```python
from build123d import *

# Parameters (mm, degrees)
BOSS_EXTRUDE2_DEPTH = 8
CUT_EXTRUDE5_DEPTH  = 18.5
BOSS_EXTRUDE7_DEPTH = 8
SKETCH9_R           = 3.15
CUT_EXTRUDE6_DEPTH  = 8
CUT_EXTRUDE8_DEPTH  = 8
BOSS_EXTRUDE8_DEPTH = 8
SKETCH14_R          = 5
CUT_EXTRUDE10_DEPTH = 10
SKETCH15_R          = 6
CUT_EXTRUDE11_DEPTH = 4
SKETCH2_R           = 3.15
CUT_EXTRUDE12_DEPTH = 48


with BuildPart() as part:
    # Sketch1 → Boss-Extrude2 (new body)
    with BuildSketch(Plane(origin=(0, 0, 0), x_dir=(1, 0, 0), z_dir=(0, 1, 0))):
        Polygon((-36.064195387, 30.19821093), (-36.064195387, 45.055140387), (-24.456215945, 60.508200645), (25.928290152, 75.028423128), (63.192701615, 49.978777876), (57.8600206, 4.654046233), (5.024212079, -12.575443702), (-26.79369062, -0.934399252), align=None)
    extrude(amount=BOSS_EXTRUDE2_DEPTH)

    # Sketch7 → Cut-Extrude5 (cut)
    with BuildSketch(Plane(origin=(0, 8, 0), x_dir=(1, 0, 0), z_dir=(0, 1, 0))):
        Polygon((-23.90080129, 101.032848336), (-57.901406204, 20.736967462), (-18.158957139, -32.533824917), (87.924213713, -9.961236853), (85.311975199, 49.315634488), align=None)
        Polygon((-40.820623888, 23.42964982), (-5.371906334, -12.019067733), (42.940552226, -17.400063196), (73.057764711, 41.083606285), (-8.197554073, 82.927487203), align=None, mode=Mode.SUBTRACT)
    extrude(amount=-CUT_EXTRUDE5_DEPTH, mode=Mode.SUBTRACT)

    # Sketch8 → Boss-Extrude7 (add)
    with BuildSketch(Plane(origin=(0, 8, 0), x_dir=(1, 0, 0), z_dir=(0, 1, 0))):
        Polygon((-8.197554073, 82.927487203), (-40.820623888, 23.42964982), (-5.371906334, -12.019067733), (42.940552226, -17.400063196), (73.057764711, 41.083606285), align=None)
        Polygon((7.41963674, 62.005546744), (-9.746922841, 64.747246038), (-32.401642497, 23.42964982), (0, -4.674812176), (46.197479834, 11.841771544), (56.025503799, 35.943618774), align=None, mode=Mode.SUBTRACT)
    extrude(amount=-BOSS_EXTRUDE7_DEPTH)

    # Sketch9 → Cut-Extrude6 (cut)
    with BuildSketch(Plane(origin=(0, 0, 0), x_dir=(-1, 0, 0), z_dir=(0, -1, 0))):
        with Locations((-28.941808693, 3.473889793)):
            Circle(SKETCH9_R)
    extrude(amount=-CUT_EXTRUDE6_DEPTH, mode=Mode.SUBTRACT)

    # Sketch10 → Cut-Extrude8 (cut)
    with BuildSketch(Plane(origin=(0, 8, 0), x_dir=(1, 0, 0), z_dir=(0, 1, 0))):
        Polygon((-51.027907223, 26.499697203), (-18.337970987, 89.979258173), (70.618900133, 64.73001084), (85.862243499, 8.329361683), (41.198193823, -31.646717715), (-23.676019088, -9.814381331), align=None)
        with BuildLine():
            Line((-33.872566493, 31.841833363), (-7.610913822, 63.637460521))
            ThreePointArc((-7.610913822, 63.637460521), (-0.606725689, 67.783190008), (7.431616747, 66.506171896))
            Line((7.431616747, 66.506171896), (48.870452229, 43.677060264))
            ThreePointArc((48.870452229, 43.677060264), (53.514897305, 39.092266426), (55.073012074, 32.754799821))
            Line((55.073012074, 32.754799821), (41.706263242, -9.064889609))
            ThreePointArc((41.706263242, -9.064889609), (33.18888877, -18.343686498), (20.602861854, -17.860296318))
            Line((20.602861854, -17.860296318), (-29.950777497, 7.924950794))
            ThreePointArc((-29.950777497, 7.924950794), (-37.823070784, 18.242703419), (-34.700474084, 30.839465332))
            Line((-34.700474084, 30.839465332), (-33.872566493, 31.841833363))
        make_face(mode=Mode.SUBTRACT)
    extrude(amount=-CUT_EXTRUDE8_DEPTH, mode=Mode.SUBTRACT)

    # Sketch12 → Boss-Extrude8 (add)
    with BuildSketch(Plane(origin=(0, 8, 0), x_dir=(1, 0, 0), z_dir=(0, 1, 0))):
        with BuildLine():
            Line((-34.700474084, 30.839465332), (-23.799416497, 10.878604368))
            Line((-23.799416497, 10.878604368), (16.273254251, -10.775107124))
            Line((16.273254251, -10.775107124), (41.706263242, -9.064889609))
            ThreePointArc((41.706263242, -9.064889609), (33.18888877, -18.343686498), (20.602861854, -17.860296318))
            Line((20.602861854, -17.860296318), (-29.950777497, 7.924950794))
            ThreePointArc((-29.950777497, 7.924950794), (-37.823070784, 18.242703419), (-34.700474084, 30.839465332))
        make_face()
    extrude(amount=-BOSS_EXTRUDE8_DEPTH)

    # Sketch14 → Cut-Extrude10 (cut)
    with BuildSketch(Plane(origin=(0, 0, 0), x_dir=(-1, 0, 0), z_dir=(0, -1, 0))):
        with Locations((-28.006293823, 31.687531628)):
            Circle(SKETCH14_R)
    extrude(amount=-CUT_EXTRUDE10_DEPTH, mode=Mode.SUBTRACT)

    # Sketch15 → Cut-Extrude11 (cut)
    with BuildSketch(Plane.XZ):
        with Locations((28.006293823, -31.687531628)):
            Circle(SKETCH15_R)
    extrude(amount=-CUT_EXTRUDE11_DEPTH, mode=Mode.SUBTRACT)

    # Sketch2 → Cut-Extrude12 (cut)
    with BuildSketch(Plane(origin=(0, 8, 0), x_dir=(1, 0, 0), z_dir=(0, 1, 0))):
        with Locations((-0.992606529, 5.023658057)):
            Circle(SKETCH2_R)
        with Locations((-23.973939823, 24.307286348)):
            Circle(SKETCH2_R)
    extrude(amount=-CUT_EXTRUDE12_DEPTH, mode=Mode.SUBTRACT)


solid = part.part
```
The listing builds one solid part. Answer for the finished solid, in the listing's coordinates (mm). A direction names the side the tool comes from. Give positions to 0.01 mm unless a question says otherwise; leave off trailing zeros. Order: outer loops, then holes, each group sorted by start corner. A loop starts at its lowest first (then second) coordinate and runs counter-clockwise, first axis right, second up. Notation, with made-up numbers: (23, 77.5) - (65, 77.5) arc R15 ccw to (65, 85.5) - close; hole circle Ø11 at (55, 51). An arc over 180 degrees is marked (long way). Answer in a Markdown table with one row per item. Add a question column.
Q1. The part is cut by section A-A (x = 29.5). Determine the outline of the cut face in (y, z).
Q2. The part is cut by section C-C (z = -20). Determine the outline of the cut face in (x, y).
Q3. Which of the six approach directions +Z, -Z, +X, -X, +Y, -Y give full straight-line access (tool end or side, diameter ignored) to faces 5 (the cylindrical face through (23.245, 1.972, -35.338)), 6 (the flat face through (48.483, 4.056, -12.138))?
Q4. The part is cut by section D-D (x = 10.5). Determine the outline of the cut face in (y, z).
Q5. Given P1, Ø1, axis at y = 6, z = -47, coming from the +X side; P2, Ø2, axis at x = 34, y = 3, coming from the -Z side; P3, Ø8, axis at x = 28.01, z = -31.69, coming from the +Y side; P4, Ø1, axis at y = 2, z = -52, coming from the +X side, each flat-ended and moving along its own axis, determine where each tip first touches the part or whether it passes through.
Q6. For a pull along X with two mould halves and no side action, classify faces 1 (the flat face through (-4.32, 4.06, 5.15)), 2 (the flat face through (27.86, 4.06, -55.25)), 3 (the flat face through (8, 0, -25)), 4 (the flat face through (24, 4, -28)) as released by +X, released by -X, zero draft, split by the parting line, or undercut.
Q7. Find the intervals of material crossed by line 1 along X through (y, z) = (3, -6); line 2 along X through (y, z) = (7.75, -30.5); line 3 along X through (y, z) = (7.75, -34.5), in increasing order. Write a range as [from, to].
Q8. The part is cut by section B-B (y = 1.5). Determine the outline of the cut face in (x, z).
Determined:
| question | item | result |
|---|---|---|
| 1 | outline | (0, -54.35) - (8, -54.35) - (8, -36.46) - (4, -36.46) - (4, -37.5) - (0, -37.5) - close; (0, -25.88) - (4, -25.88) - (4, -26.92) - (8, -26.92) - (8, -6.57) - (0, -6.57) - close; (0, -0.37) - (8, -0.37) - (8, 19.35) - (0, 19.35) - close |
| 2 | outline | (-38.08, 0) - (51, 0) - (51, 8) - (-38.08, 8) - close |
| 3 | face 5 | -Y |
| 3 | face 6 | +Z, +X, +Y, -Y |
| 4 | outline | (0, -64.82) - (8, -64.82) - (8, 12.71) - (0, 12.71) - close |
| 5 | P1 | stops at x = 43.75 |
| 5 | P2 | stops at z = -52.42 |
| 5 | P3 | passes through |
| 5 | P4 | stops at x = 34.67 |
| 6 | face 1 | released by -X |
| 6 | face 2 | released by +X |
| 6 | face 3 | zero draft |
| 6 | face 4 | undercut |
| 7 | line 1 | x = [-26.18, -3.99], [2, 27.06], [30.82, 46.52] |
| 7 | line 2 | x = [-34.97, 23.15], [32.86, 54.35] |
| 7 | line 3 | x = [-31.68, 23.87], [32.14, 55.01] |
| 8 | outline | (-34.7, -30.84) - (-7.61, -63.64) arc R12 ccw to (7.43, -66.51) - (48.87, -43.68) arc R12 ccw to (55.07, -32.75) - (41.71, 9.06) arc R15 ccw to (20.6, 17.86) - (-29.95, -7.92) arc R15 ccw to start; hole circle Ø6.3 at (-23.97, -24.31); hole circle Ø6.3 at (-0.99, -5.02); hole circle Ø12 at (28.01, -31.69); hole circle Ø6.3 at (28.94, -3.47) |
